```python
from build123d import *

# Parameters (mm, degrees)
SKETCH4_R           = 4
BOSS_EXTRUDE4_DEPTH = 3.2
BOSS_EXTRUDE6_START = -3.2
BOSS_EXTRUDE6_DEPTH = 3.2
CIRPATTERN3_COUNT   = 7
CIRPATTERN3_ANGLE   = 111


with BuildPart() as part:
    # Sketch4 → Boss-Extrude4 (new body)
    with BuildSketch(Plane.XY):
        with BuildLine():
            Line((21.067900641, 33.325122256), (19.993019925, 53.547837419))
            ThreePointArc((19.993019925, 53.547837419), (14.939517656, 58.282084655), (10.002153079, 53.426838719))
            Line((10.002153079, 53.426838719), (9.098366441, 33.414868889))
            ThreePointArc((9.098366441, 33.414868889), (14.90552884, 9.682805465), (21.067900641, 33.325122256))
        make_face()
        with Locations((15, 22.282451301)):
            Circle(SKETCH4_R, mode=Mode.SUBTRACT)
    extrude(amount=BOSS_EXTRUDE4_DEPTH)

    # Sketch6 → Boss-Extrude6 (add)
    with BuildSketch(Plane.XY.offset(3.2).offset(BOSS_EXTRUDE6_START)):
        with BuildLine():
            Line((27.587419579, 21.71954071), (30.726886196, 20.216575064))
            ThreePointArc((30.726886196, 20.216575064), (31.03657327, 19.658315603), (30.545192773, 19.250755893))
            Line((30.545192773, 19.250755893), (27.114578574, 18.81878475))
            ThreePointArc((27.114578574, 18.81878475), (27.435866455, 20.255328827), (27.587419579, 21.71954071))
        make_face()
    boss_extrude6 = extrude(amount=BOSS_EXTRUDE6_DEPTH)

    # CirPattern3: Boss-Extrude6 ×7 about axis
    cirpattern3_axis = Axis((15, 22.282451301, 0), (0, 0, -1))
    for i in range(1, CIRPATTERN3_COUNT):
        add(boss_extrude6.rotate(cirpattern3_axis, i * CIRPATTERN3_ANGLE / (CIRPATTERN3_COUNT - 1)))


solid = part.part
```
Input: part model. Units: mm. Frame: model coordinates. A direction names the side the tool comes from. Give positions to 0.01 mm unless a question says otherwise; leave off trailing zeros. Order: outer loops, then holes, each group sorted by start corner. A loop starts at its lowest first (then second) coordinate and runs counter-clockwise, first axis right, second up. Notation, with made-up numbers: M 45,18 L 67,18 A7 ccw 67,25 Z; hole C -6.5,87.25 d7. An arc over 180 degrees is marked long. One line per question, with ' | ' between items.
1) Ray query, L1, parallel to Y at x = 14.75, z = 2.9; L2, parallel to X at y = 9.5, z = 0.95; L3, parallel to X at y = 20.5, z = 1.35. Return the intervals inside material, ascending.
Filled in:
L1: y = 9.68 to 18.29, 26.27 to 58.28 | L2: x = 6.76 to 8.66, 11.08 to 13.77, 15.09 to 17.84, 19.75 to 21.99 | L3: x = 2.53 to 11.42, 18.58 to 30.13
2) Access query for faces 4 (the face through (21.932, 9.895, 1.578)), 5 (the face through (17.643, 8.335, 1.578)), 6 (the face through (7.006, 10.512, 1.578)), 7 (the face through (28.854, 19.038, 1.578)), 8 (the face through (17, 27, 3.2)). Directions: +Z, -Z, +X, -X, +Y, -Y. A direction counts if a zero-diameter tool reaches every point of the face in a straight line with its end or side. Return the directions, or none.
Filled in:
face 4: +Z, -Z | face 5: +Z, -Z, -Y | face 6: +Z, -Z, -X | face 7: +Z, -Z, +X | face 8: +Z, +X, -X, +Y, -Y
3) Section B-B on x = 23.75. Output: boundary loops of the cut face in (y, z), and give its area (3 significant figures).
Filled in:
outline: M 11.56,0 L 31.35,0 L 31.35,3.2 L 11.56,3.2 Z | area: 63.3 mm2
4) Draft query along X for faces 1 (the face through (15.047, 58.282, 1.578)), 2 (the face through (13.08, 8.22, 1.58)), 3 (the face through (20.54, 43.29, 1.58)). Return one class per face: pulls with the +X half, pulls with the -X half, needs draft (parallel to the pull), parting line crosses it, or undercut.
Filled in:
face 1: parting line crosses it | face 2: undercut | face 3: pulls with the +X half
5) Contact query for a flat-ended pin moving along its axis: P1, Ø10, axis at x = 6, y = 32.5, coming from the -Z side. Output: stop coordinate, or through.
Filled in:
P1: stops at z = 0
6) Section C-C on y = 27. Output: boundary loops of the cut face in (x, z).
Filled in:
outline: M 3.32,0 L 26.68,0 L 26.68,3.2 L 3.32,3.2 Z
